Check sheet for the drawn part. Datum: minimum x, y, z corner. Units: mm. Give positions to 0.01 mm unless a question says otherwise; leave off trailing zeros. Loops run counter-clockwise (first coordinate to the right, second up) from the corner with the lowest first, then second, coordinate; pieces in that order, holes last. Notation, with made-up numbers: (26.25, 31.5) - (39.25, 31.5) arc R14 cw to (39.25, 36.5) - close; hole circle Ø2 at (-3, 17). An arc over 180 degrees is marked (long way). Answer in a Markdown table with one row per item.
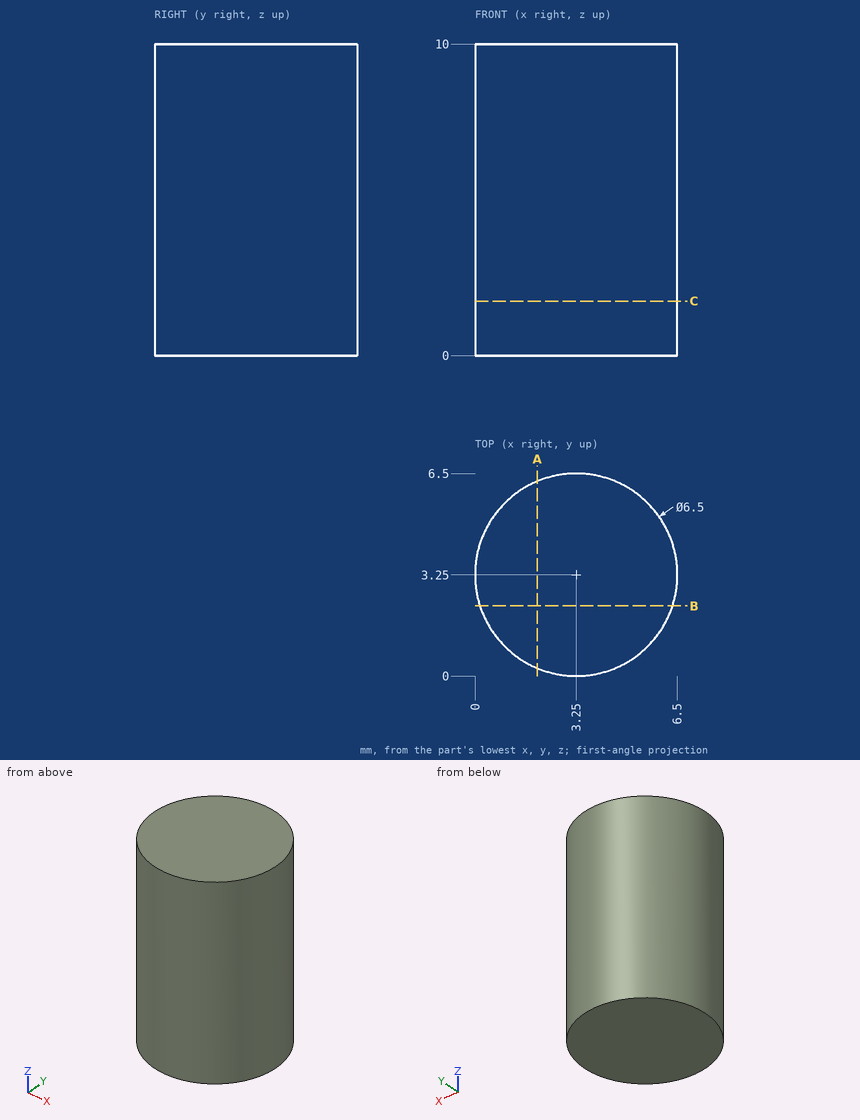
Q1. Sectioned sample at C-C (z = 1.75). Record the cut outline in (x, y), and give its area (3 significant figures).
Completed:
| item | result |
|---|---|
| outline | circle Ø6.5 at (3.25, 3.25) |
| area | 33.2 mm^2 |
Q2. Sectioned sample at A-A (x = 2). Record the cut outline in (y, z).
Completed:
| item | result |
|---|---|
| outline | (0.25, 0) - (6.25, 0) - (6.25, 10) - (0.25, 10) - close |
Q3. Thickness scan on line 1 (X direction, y = 2.75, z = 5.5); line 2 (X direction, y = 6.25, z = 5.5); line 3 (Y direction, x = 0.75, z = 7). Record the ranges inside material, lowest first.
Completed:
| item | result |
|---|---|
| line 1 | 0.04 to 6.46 |
| line 2 | 2 to 4.5 |
| line 3 | 1.17 to 5.33 |
Q4. Sectioned sample at B-B (y = 2.25). Record the cut outline in (x, z), and give its area (3 significant figures).
Completed:
| item | result |
|---|---|
| outline | (0.16, 0) - (6.34, 0) - (6.34, 10) - (0.16, 10) - close |
| area | 61.8 mm^2 |
Q5. Go/stop test with flat-tipped pins: P1, Ø1, axis at y = 4.5, z = 7.5, coming from the +X side; P2, Ø2, axis at x = 1, z = 8.5, coming from the +Y side; P3, Ø1.5, axis at x = 5, z = 3.5, coming from the -Y side. Record where each tip stops, or that it passes through.
Completed:
| item | result |
|---|---|
| P1 | x = 6.41 |
| P2 | y = 6.25 |
| P3 | y = 0.16 |
